For this review, take the finished solid that the model builds, in its own axes (mm). Give positions to 0.01 mm unless a question says otherwise; leave off trailing zeros. Loops run counter-clockwise (first coordinate to the right, second up) from the corner with the lowest first, then second, coordinate; pieces in that order, holes last.
```python
from build123d import *

# Parameters (mm, degrees)
F1_DEPTH = 2


with BuildPart() as f1:
    # F0 (on Front) → F1 (new body)
    with BuildSketch(Plane.XZ):
        Polygon((0.437443, 5), (0, 0), (17, 0), (17, 2), (283, 2), (283, 0), (300, 0), (299.562557, 5), (294.562557, 5), (293.68767, 15), (298.68767, 15), (298.250227, 20), (283, 20), (283, 10), (281, 10), (281, 16), (266.5, 16), (266.5, 10), (264.5, 10), (264.5, 16), (250, 16), (250, 10), (248, 10), (248, 16), (233.5, 16), (233.5, 10), (231.5, 10), (231.5, 16), (217, 16), (217, 10), (215, 10), (215, 16), (200.5, 16), (200.5, 10), (198.5, 10), (198.5, 16), (184, 16), (184, 10), (182, 10), (182, 16), (167.5, 16), (167.5, 10), (165.5, 10), (165.5, 16), (151, 16), (151, 10), (149, 10), (149, 16), (134.5, 16), (134.5, 10), (132.5, 10), (132.5, 16), (118, 16), (118, 10), (116, 10), (116, 16), (101.5, 16), (101.5, 10), (99.5, 10), (99.5, 16), (85, 16), (85, 10), (83, 10), (83, 16), (68.5, 16), (68.5, 10), (66.5, 10), (66.5, 16), (52, 16), (52, 10), (50, 10), (50, 16), (35.5, 16), (35.5, 10), (33.5, 10), (33.5, 16), (19, 16), (19, 10), (17, 10), (17, 20), (1.749773, 20), (1.31233, 15), (6.31233, 15), (5.437443, 5), align=None)
    extrude(amount=F1_DEPTH)


solid = f1.part
```
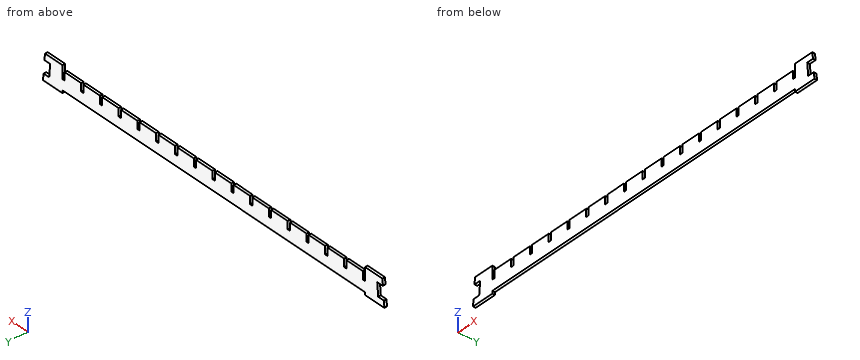
Item 1: Take a section at A-A on x = 128.5. Give the boundary of the cut face in (y, z), and give its area (3 significant figures).
Answer:
outline: (-2, 2) - (0, 2) - (0, 16) - (-2, 16) - close
area: 28.0 mm2
Item 2: Clearance check with flat-ended pins moving along their axes: pin 1 Ø1 at (y, z) = (-0.5, 4.5) entering from +X; pin 2 Ø0.6 at (x, y) = (216, -1.5) entering from +Z; pin 3 Ø1 at (y, z) = (-0.5, 13.5) entering from +X. State where each tip first meets the part, or that it passes through.
Answer:
pin 1: stops at x = 299.65
pin 2: stops at z = 10
pin 3: stops at x = 293.86
Item 3: For L1, parallel to X at y = -1.6, z = 17.5; L2, parallel to Z at x = 56, y = -0.35; L3, parallel to X at y = -0.85, z = 18.25, list the stretches that pass through material, from the lowest coordinate up.
Answer:
L1: x = 1.53 to 17, 283 to 298.47
L2: z = 2 to 16
L3: x = 1.6 to 17, 283 to 298.4
